Can you work these out from the model? Positions are in its coordinate system, mm. A direction names the side the tool comes from. Give positions to 0.01 mm unless a question says otherwise; leave off trailing zeros. Order: outer loops, then holes, each group sorted by start corner. A loop starts at its lowest first (then second) coordinate and runs counter-clockwise, first axis right, second up.
```python
from build123d import *

# Parameters (mm, degrees)
SKETCH1_R           = 1.5
BOSS_EXTRUDE4_DEPTH = 6


with BuildPart() as part:
    # Sketch1 → Boss-Extrude4 (new body)
    with BuildSketch(Plane(origin=(0, 0, 0), x_dir=(1, 0, 0), z_dir=(0, 1, 0))):
        with BuildLine():
            Line((12, 0), (6, 150))
            ThreePointArc((6, 150), (0, 156), (-6, 150))
            Line((-6, 150), (-12, 0))
            Line((-12, 0), (-6, -50))
            ThreePointArc((-6, -50), (0, -56), (6, -50))
            Line((6, -50), (12, 0))
        make_face()
        with Locations(Location((0, 0, 0), (0, 0, 270))):
            Circle(SKETCH1_R, mode=Mode.SUBTRACT)
        with BuildLine():
            Line((-0.714871324, -44.042738969), (-4.673707022, -11.05244148))
            ThreePointArc((-4.673707022, -11.05244148), (0, -12), (4.673707022, -11.05244148))
            Line((4.673707022, -11.05244148), (0.714871324, -44.042738969))
            ThreePointArc((0.714871324, -44.042738969), (0, -44), (-0.714871324, -44.042738969))
        make_face(mode=Mode.SUBTRACT)
        with BuildLine():
            Line((0.23980823, 144.004794248), (5.574944726, 10.626381854))
            ThreePointArc((5.574944726, 10.626381854), (0, 12), (-5.574944726, 10.626381854))
            Line((-5.574944726, 10.626381854), (-0.23980823, 144.004794248))
            ThreePointArc((-0.23980823, 144.004794248), (0, 144), (0.23980823, 144.004794248))
        make_face(mode=Mode.SUBTRACT)
        with Locations(Location((0, 150, 0), (0, 0, 270))):
            Circle(SKETCH1_R, mode=Mode.SUBTRACT)
        with Locations(Location((0, -50, 0), (0, 0, 270))):
            Circle(SKETCH1_R, mode=Mode.SUBTRACT)
    extrude(amount=BOSS_EXTRUDE4_DEPTH)


solid = part.part
```
1) Suppose I cut it at B-B (y = 4). Please give me the cut outline in (x, z), and give its area (3 significant figures).
2) Suppose I cut it at C-C (x = -9.25). Please give me the cut outline in (y, z), and give its area (3 significant figures).
3) Which directions (+Z, -Z, +X, -X, +Y, -Y) give clear straight access to the entire face, cutting with the end or side of a thin tool? Please do faces 1 (the face through (2.72, 2.96, 27.32)), 2 (the face through (9, 3, 25)).
4) We'd pull the mould along X, two halves only. Please class faces 3 (the face through (5, 6, -51)), 4 (the face through (-2.667, 2.958, 27.779)), 5 (the face through (-8.96, 2.96, -76.05)), 6 (the face through (9.04, 2.96, -73.95)): +X half, -X half, draft (parallel to the pull), parting line (faces both ways), or undercut.
5) If I drill on line 1 (X direction, y = 1.9, z = 0); line 2 (X direction, y = 3.3, z = -150), over which ranges is the centre line in solid material (lowest first)?
6) Suppose I cut it at A-A (z = -34.5). Please give me the cut outline in (x, y), and give its area (3 significant figures).
7) Suppose I cut it at D-D (x = 9.5). Please give me the cut outline in (y, z), and give its area (3 significant figures).
8) I'm going to push flat-ended pins straight in: pin 1 Ø1.5 at (x, y) = (-1, 1.5) entering from -Z; pin 2 Ø2.5 at (x, z) = (0, 50) entering from -Y; pin 3 Ø1.5 at (y, z) = (2, -57.5) entering from +X. Where does each tip first touch, or does it pass through?
Results:
1. outline: (-12, 0) - (-6, -150) arc R6 ccw to (6, -150) - (12, 0) - (6, 50) arc R6 ccw to (-6, 50) - close; hole (-5.57, -10.63) - (-0.24, -144) arc R6 cw to (0.24, -144) - (5.57, -10.63) arc R12 cw to start; hole (-4.67, 11.05) arc R12 cw to (4.67, 11.05) - (0.71, 44.04) arc R6 cw to (-0.71, 44.04) - close; hole circle Ø3 at (0, -150); hole circle Ø3 at (0, 0); hole circle Ø3 at (0, 50)
1. area: 2,750 mm2
2. outline: (0, -68.75) - (6, -68.75) - (6, 22.92) - (0, 22.92) - close
2. area: 550 mm2
3. face 1: +Y, -Y
3. face 2: +Z, +X, +Y, -Y
4. face 3: draft
4. face 4: undercut
4. face 5: -X half
4. face 6: +X half
5. line 1: x = -12 to -1.5, 1.5 to 12
5. line 2: x = -6 to -1.5, 1.5 to 6
6. outline: (-10.62, 0) - (-4.62, 0) - (-4.62, 6) - (-10.62, 6) - close; (4.62, 0) - (10.62, 0) - (10.62, 6) - (4.62, 6) - close
6. area: 72.0 mm2
7. outline: (0, -62.5) - (6, -62.5) - (6, 20.83) - (0, 20.83) - close
7. area: 500 mm2
8. pin 1: stops at z = -155.99
8. pin 2: passes through
8. pin 3: stops at x = 9.73
